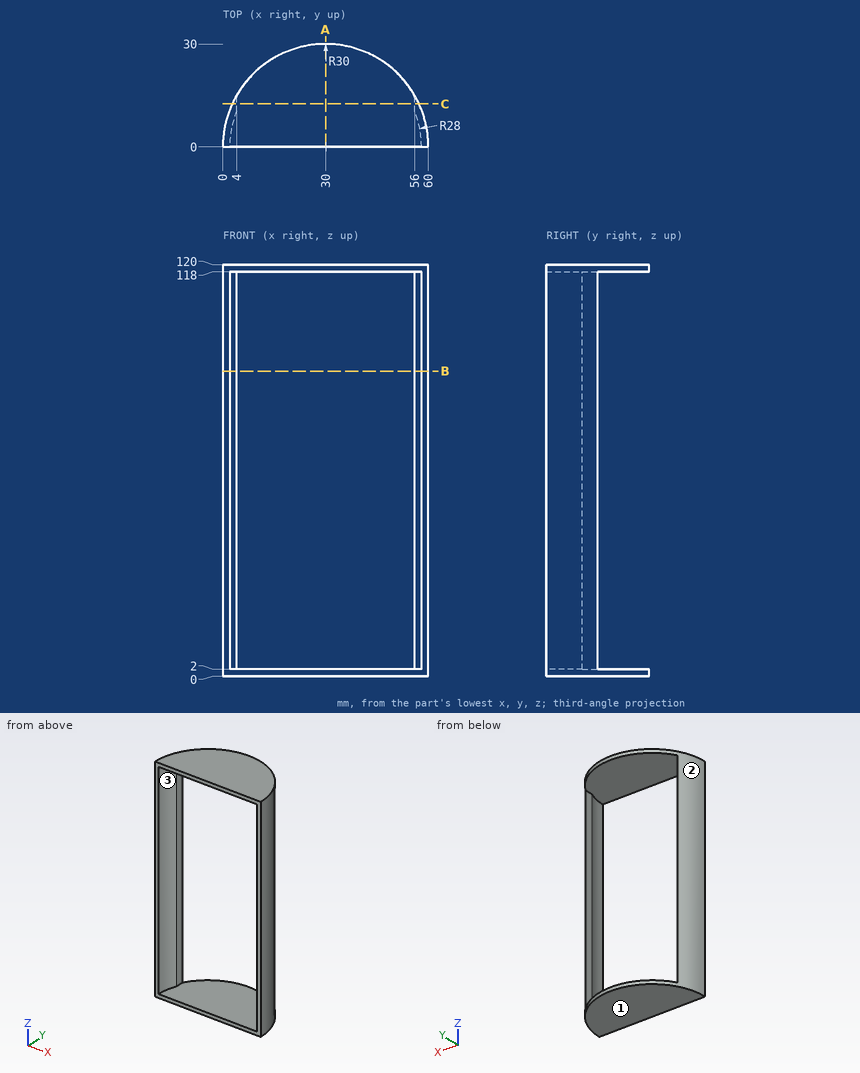
Job drawing, mm, ordinate dimensions from the low corner. One solid piece. Round coordinates to 2 decimals unless told otherwise and drop trailing zeros. Loops run counter-clockwise (first coordinate to the right, second up) from the corner with the lowest first, then second, coordinate; pieces in that order, holes last. Notation, with made-up numbers: M 30,35 L 55,35 A27 cw 55,63 Z; hole C 5.25,35 d3. An arc over 180 degrees is marked long. One line per question, with ' | ' between items. Start each with the question number.
Item 1: Pin check, flat tips, straight feed: pin 1 Ø6 at (y, z) = (16.5, 30.5) entering from -X; pin 2 Ø15 at (x, y) = (39.5, 7.5) entering from -Z; pin 3 Ø3 at (y, z) = (8.5, 97) entering from -X; pin 4 Ø5 at (x, z) = (7, 87.5) entering from -Y. Stop position of each tip, or through.
Item 2: Cut at C-C, the plane y = 12.5. Write the cut outline in (x, z).
Item 3: Cut at A-A, the plane x = 30. Write the cut outline in (y, z).
Item 4: Two-plate mould, pull along X, no slides. Class the marked faces 1, 2 and 3: pulls with the +X half, pulls with the -X half, needs draft (parallel to the pull), parting line crosses it, or undercut.
Item 5: Cut at B-B, the plane z = 89. Write the cut outline in (x, y).
Item 6: Wall check: line 1 (Z direction, x = 37, y = 26.75); line 2 (X direction, y = 4, z = 6); line 3 (X direction, y = 2.5, z = 59.5). Give the ranges that are in metal, low to high.
Responses:
1) pin 1: stops at x = 3.21 | pin 2: stops at z = 0 | pin 3: stops at x = 0.83 | pin 4: passes through
2) outline: M 2.73,0 L 57.27,0 L 57.27,120 L 2.73,120 Z; hole M 4,2 L 56,2 L 56,118 L 4,118 Z
3) outline: M 0,0 L 30,0 L 30,2 L 0,2 Z; M 0,118 L 30,118 L 30,120 L 0,120 Z
4) face 1: needs draft | face 2: parting line crosses it | face 3: undercut
5) outline: M 0,0 L 2,0 A28 cw 4,10.39 L 4,14.97 A30 ccw Z; M 56,10.39 A28 cw 58,0 L 60,0 A30 ccw 56,14.97 Z
6) line 1: z = 0 to 2, 118 to 120 | line 2: x = 0.27 to 2.29, 57.71 to 59.73 | line 3: x = 0.1 to 2.11, 57.89 to 59.9
